```python
from build123d import *

# Parameters (mm, degrees)
F0_W     = 600
F0_H     = 600
F1_DEPTH = 50.8
F3_W     = 70
F3_H     = 70
F4_DEPTH = 400
F5_COUNT = 4


with BuildPart() as f1:
    # F0 (on Top) → F1 (new body)
    with BuildSketch(Plane.XY):
        Rectangle(F0_W, F0_H)
    extrude(amount=F1_DEPTH)

    # F3 (on Top) → F4 (join)
    with BuildSketch(Plane.XY):
        with Locations((-250, -250)):
            Rectangle(F3_W, F3_H)
    extrude(amount=-F4_DEPTH)

    # F5: F1 ×4 about axis
    f5_axis = Axis((0, 0, -387.7218663692), (0, 0, 1))


with BuildPart() as f1_1:
    add(f1.part)
    for i in range(1, F5_COUNT):
        add(f1.part.rotate(f5_axis, i * 360 / F5_COUNT))


solid = f1_1.part
```
Geometry: final body of the model. Coordinates: model frame, mm. A direction names the side the tool comes from. Round coordinates to 2 decimals unless told otherwise and drop trailing zeros. Order: outer loops, then holes, each group sorted by start corner. A loop starts at its lowest first (then second) coordinate and runs counter-clockwise, first axis right, second up. Notation, with made-up numbers: (35, 30.5) - (55, 30.5) arc R22 ccw to (55, 54.5) - close; hole circle Ø3 at (44.5, 78). An arc over 180 degrees is marked (long way). Write item = value, one per line. Start each with the question number.
Q1. Ray query, line 1 (X direction, y = -233.5, z = -227); line 2 (Z direction, x = 206, y = -234.5). Return the intervals inside material, ascending. Write a range as from..to.
Q2. Access query for faces 1 (the flat face through (250, -285, -197)), 2 (the flat face through (-250, 285, -197)), 3 (the flat face through (285, -250, -197)). Directions: +Z, -Z, +X, -X, +Y, -Y. A direction counts if a zero-diameter tool reaches every point of the face in a straight line with its end or side. Return the directions, or none.
Q3. Pin query (flat end, axial travel): pin 1 (21 mm diameter, centred on x = -256.5, z = -281, fed in from -Y); pin 2 (1.5 mm diameter, centred on y = -214, z = -203, fed in from -X); pin 3 (21 mm diameter, centred on y = 266, z = -144, fed in from -X); pin 4 (21 mm diameter, centred on y = 253, z = -218, fed in from +X). Return the tip coordinate at first contact, or that it passes through.
Q4. Cut plane D-D on y = -6. Return the cut outline in (x, z).
Q5. Cut plane B-B on x = 259.5. Return the cut outline in (y, z).
Q6. Cut plane A-A on z = -137. Return the cut outline in (x, y), and give its area (3 significant figures).
Outcome:
q1.line_1 = -285..-215, 215..285
q1.line_2 = 0..50.8
q2.face_1 = -Z, +X, -X, -Y
q2.face_2 = -Z, +X, -X, +Y
q2.face_3 = -Z, +X, +Y, -Y
q3.pin_1 = -285
q3.pin_2 = through
q3.pin_3 = -285
q3.pin_4 = 285
q4.outline = (-300, 0) - (300, 0) - (300, 50.8) - (-300, 50.8) - close
q5.outline = (-300, 0) - (-285, 0) - (-285, -400) - (-215, -400) - (-215, 0) - (215, 0) - (215, -400) - (285, -400) - (285, 0) - (300, 0) - (300, 50.8) - (-300, 50.8) - close
q6.outline = (-285, -285) - (-215, -285) - (-215, -215) - (-285, -215) - close; (-285, 215) - (-215, 215) - (-215, 285) - (-285, 285) - close; (215, -285) - (285, -285) - (285, -215) - (215, -215) - close; (215, 215) - (285, 215) - (285, 285) - (215, 285) - close
q6.area = 19,600 mm^2
